Source: CAD feature listing. Evaluate the final solid. Frame: model axes, mm. A direction names the side the tool comes from. Give positions to 0.01 mm unless a question says otherwise; leave off trailing zeros. Write each loop counter-clockwise with the first axis right and the second up, starting at its lowest first coordinate (ties: lowest second). Pieces come first, ordered by that corner, then holes. Notation, with made-up numbers: (-8.75, 77) - (14.25, 77) arc R23 cw to (14.25, 108) - close; hole circle Ø4 at (87, 58.25). An arc over 180 degrees is marked (long way). Answer as a JSON object with one key per item and string values. Group by question number.
from build123d import *

# Parameters (mm, degrees)
SKETCH1_R           = 2.5
BOSS_EXTRUDE1_DEPTH = 8
SKETCH2_R           = 1.5
CUT_EXTRUDE1_DEPTH  = 77.487541414
FILLET1_R           = 10
SKETCH3_R           = 6
CUT_EXTRUDE2_DEPTH  = 77.487541414


with BuildPart() as part:
    # Sketch1 → Boss-Extrude1 (new body)
    with BuildSketch(Plane.XY):
        with BuildLine():
            Line((0, -19), (30, -19))
            Line((30, -19), (64.201367261, 15.201367261))
            Line((64.201367261, 15.201367261), (58.615223689, 20.787510832))
            Line((58.615223689, 20.787510832), (31.745166004, -6.082546853))
            Line((31.745166004, -6.082546853), (17.320187668, 8.342431483))
            Line((17.320187668, 8.342431483), (44.190245353, 35.212489168))
            Line((44.190245353, 35.212489168), (38.604101782, 40.798632739))
            Line((38.604101782, 40.798632739), (16.805469042, 19))
            Line((16.805469042, 19), (0, 19))
            ThreePointArc((0, 19), (-19, 0), (0, -19))
        make_face()
        Circle(SKETCH1_R, mode=Mode.SUBTRACT)
    extrude(amount=BOSS_EXTRUDE1_DEPTH)

    # Sketch2 → Cut-Extrude1 (cut, through all)
    with BuildSketch(Plane.XY.offset(8)):
        with Locations((38.878105659, 35.574881393)):
            Circle(SKETCH2_R)
        with Locations((58.977615915, 15.475371138)):
            Circle(SKETCH2_R)
    extrude(amount=-CUT_EXTRUDE1_DEPTH, mode=Mode.SUBTRACT)

    # Fillet1
    fillet1_edges = [part.edges().sort_by_distance(p)[0] for p in [
        (30, -19, 4),
        (16.805469042, 19, 4),
    ]]
    fillet(fillet1_edges, radius=FILLET1_R)

    # Sketch3 → Cut-Extrude2 (cut, through all)
    with BuildSketch(Plane.XY.offset(8)):
        Circle(SKETCH3_R)
        Polygon((38.604101782, 40.798632739), (64.201367261, 15.201367261), (57.130299449, 8.130299449), (31.53303397, 33.727564928), align=None)
    extrude(amount=-CUT_EXTRUDE2_DEPTH, mode=Mode.SUBTRACT)


solid = part.part
Q1. Draft query along Y for faces 4 (the flat face through (25.716, 27.911, 3.944)), 5 (the cylindrical face through (-19, 0, 4)), 6 (the cylindrical face through (-6, 0, 4)). Return one class per face: released by +Y, released by -Y, zero draft, split by the parting line, or undercut.
Q2. Section B-B on z = 4.25. Return the cut outline in (x, y), then the cut area to 3 significant figures.
Q3. Section C-C on x = 25. Return the cut outline in (y, z).
Q4. Section D-D on x = -13.5. Return the cut outline in (y, z), then the cut area to 3 significant figures.
Q5. Section A-A on y = 3. Return the cut outline in (x, z).
Q6. Ray query, probe 1 along Y at (x, z) = (0, 5.5); probe 2 along X at (y, z) = (-5, 3.5); probe 3 along X at (y, z) = (-0.5, 4.25). Return the intervals inside material, ascending. Write a range as [from, to].
Q7. Reachability of faces 1 (the flat face through (24.63, 1.03, 3.94)), 2 (the flat face through (34.365, 30.895, 4.056)), 3 (the flat face through (6, 19, 4)) from +Z, -Z, +X, -X, +Y, -Y: full face, straight path, thin tool, end or side. Return the list, or none.
Q8. First-contact query: pin 1 Ø1 at (x, z) = (36, 7) entering from +Y; pin 2 Ø4 at (x, z) = (8, 5) entering from +Y; pin 3 Ø1 at (y, z) = (14.5, 6) entering from -X. Flat tips, straight axial feed; report the tip coordinate or a pass-through.
Taken from the geometry:
{
 "1": {"face 4": "released by +Y", "face 5": "split by the parting line", "face 6": "undercut"},
 "2": {"outline": "(0, -19) - (25.86, -19) arc R10 ccw to (32.93, -16.07) - (57.13, 8.13) - (51.54, 13.72) - (31.75, -6.08) - (17.32, 8.34) - (37.12, 28.14) - (31.53, 33.73) - (19.73, 21.93) arc R10 cw to (12.66, 19) - (0, 19) arc R19 ccw to start; hole circle Ø12 at (0, 0)", "area": "1,840 mm²"},
 "3": {"outline": "(-19, 0) - (0.66, 0) - (0.66, 8) - (-19, 8) - close; (16.02, 0) - (27.19, 0) - (27.19, 8) - (16.02, 8) - close"},
 "4": {"outline": "(-13.37, 0) - (13.37, 0) - (13.37, 8) - (-13.37, 8) - close", "area": "214 mm²"},
 "5": {"outline": "(-18.76, 0) - (-5.2, 0) - (-5.2, 8) - (-18.76, 8) - close; (5.2, 0) - (22.66, 0) - (22.66, 8) - (5.2, 8) - close; (40.83, 0) - (52, 0) - (52, 8) - (40.83, 8) - close"},
 "6": {"probe 1": "y = [-19, -6], [6, 19]", "probe 2": "x = [-18.33, -3.32], [3.32, 30.66], [32.83, 44]", "probe 3": "x = [-18.99, -5.98], [5.98, 26.16], [37.33, 48.5]"},
 "7": {"face 1": "+Z, -Z", "face 2": "+Z, -Z, +X, +Y", "face 3": "+Z, -Z, -X, +Y"},
 "8": {"pin 1": "stops at y = 29.76", "pin 2": "stops at y = 19", "pin 3": "stops at x = -12.85"}
}
